Part model, mm, in its own coordinate system. A direction names the side the tool comes from. Coordinates: 2 decimals unless noted, no trailing zeros. Order: outer loops, then holes, each group sorted by start corner. A loop starts at its lowest first (then second) coordinate and runs counter-clockwise, first axis right, second up.
from build123d import *

# Parameters (mm, degrees)
BOSS_EXTRUDE1_DEPTH          = 8
CUT_EXTRUDE1_DEPTH           = 3
F_4_0_4_DIAMETER_HOLE1_D     = 4
F_4_0_4_DIAMETER_HOLE1_DEPTH = 8
FILLET1_R                    = 3
FILLET2_R                    = 5
FILLET3_R                    = 11
FILLET4_R                    = 13


with BuildPart() as part:
    # Sketch1 → Boss-Extrude1 (new body)
    with BuildSketch(Plane.XY.offset(13)):
        with BuildLine():
            Line((-15, 5), (-15, 20))
            ThreePointArc((-15, 20), (-20, 25), (-25, 20))
            Line((-25, 20), (-25, -5))
            Line((-25, -5), (0, -5))
            ThreePointArc((0, -5), (5, 0), (0, 5))
            Line((0, 5), (-15, 5))
        make_face()
    extrude(amount=-BOSS_EXTRUDE1_DEPTH)

    # Sketch2 → Cut-Extrude1 (cut)
    with BuildSketch(Plane.XY.offset(13)):
        with BuildLine():
            Line((-23, 20), (-23, -3))
            Line((-23, -3), (0, -3))
            ThreePointArc((0, -3), (3, 0), (0, 3))
            Line((0, 3), (-17, 3))
            Line((-17, 3), (-17, 20))
            ThreePointArc((-17, 20), (-20, 23), (-23, 20))
        make_face()
    extrude(amount=-CUT_EXTRUDE1_DEPTH, mode=Mode.SUBTRACT)

    # Ø4.0 (4) Diameter Hole1
    with Locations(Plane(origin=(0, 0, 5), x_dir=(-1, 0, 0), z_dir=(0, 0, -1))):
        with Locations((20, 20), (20, 0), (0, 0)):
            Hole(F_4_0_4_DIAMETER_HOLE1_D / 2, depth=F_4_0_4_DIAMETER_HOLE1_DEPTH)

    # Fillet1
    fillet1_edges = [part.edges().sort_by_distance(p)[0] for p in [
        (-23, -3, 11.5),
    ]]
    fillet(fillet1_edges, radius=FILLET1_R)

    # Fillet2
    fillet2_edges = [part.edges().sort_by_distance(p)[0] for p in [
        (-25, -5, 9),
    ]]
    fillet(fillet2_edges, radius=FILLET2_R)

    # Fillet3
    fillet3_edges = [part.edges().sort_by_distance(p)[0] for p in [
        (-15, 5, 9),
    ]]
    fillet(fillet3_edges, radius=FILLET3_R)

    # Fillet4
    fillet4_edges = [part.edges().sort_by_distance(p)[0] for p in [
        (-17, 3, 11.5),
    ]]
    fillet(fillet4_edges, radius=FILLET4_R)


solid = part.part
Q1. Which spindle directions (+Z, -Z, +X, -X, +Y, -Y) get a long thin tool onto all of the face, cutting with end or side? Do faces 5 (the face through (-10, -5, 9)), 6 (the face through (-13.293, 6.909, 11.479)), 7 (the face through (-2, 5, 9)). Say none if no direction does.
Results list:
face 5: +Z, -Z, +X, -X, -Y
face 6: +Z
face 7: +Z, -Z, +X, +Y
Q2. Mould opens along X. For faces 1 (the face through (-16, 7, 10)), 2 (the face through (-14, 7, 5)), 3 (the face through (5, 0, 9)), 4 (the face through (-2, 3, 12)) say: pulls with the +X half, pulls with the -X half, needs draft (parallel to the pull), parting line crosses it, or undercut.
Results list:
face 1: undercut
face 2: needs draft
face 3: pulls with the +X half
face 4: undercut
Q3. Cut at A-A on z = 8.5. Write the cut outline in (x, y).
Results list:
outline: (-25, 0) arc R5 ccw to (-20, -5) - (0, -5) arc R5 ccw to (0, 5) - (-4, 5) arc R11 cw to (-15, 16) - (-15, 20) arc R5 ccw to (-25, 20) - close; hole circle Ø4 at (-20, 0); hole circle Ø4 at (-20, 20); hole circle Ø4 at (0, 0)
Q4. Cut at B-B on x = -19. Write the cut outline in (y, z).
Results list:
outline: (-5, 5) - (-1.73, 5) - (-1.73, 10) - (-3, 10) - (-3, 13) - (-5, 13) - close; (1.73, 5) - (18.27, 5) - (18.27, 10) - (1.73, 10) - close; (21.73, 5) - (24.9, 5) - (24.9, 13) - (22.83, 13) - (22.83, 10) - (21.73, 10) - close
Q5. Cut at D-D on y = 9.5. Write the cut outline in (x, z).
Results list:
outline: (-25, 5) - (-12.87, 5) - (-12.87, 13) - (-15.26, 13) - (-15.26, 10) - (-23, 10) - (-23, 13) - (-25, 13) - close
Q6. Pin check, flat tips, straight feed: pin 1 Ø2.5 at (y, z) = (9.5, 11) entering from +X; pin 2 Ø4.5 at (x, y) = (-20, 20) entering from +Z; pin 3 Ø4.5 at (y, z) = (18, 10) entering from +X. Stop position of each tip, or through.
Results list:
pin 1: stops at x = -11.81
pin 2: stops at z = 10
pin 3: stops at x = -15
Q7. Wall check: line 1 along Y through (x, z) = (-20, 7.9); line 2 along Y through (x, z) = (-1.25, 12.75); line 3 along X through (y, z) = (21.5, 11). Give the ranges that are in metal, low to high.
Results list:
line 1: y = -5 to -2, 2 to 18, 22 to 25
line 2: y = -5 to -3, 3 to 5
line 3: x = -24.77 to -22.6, -17.4 to -15.23
Q8. Cut at C-C on z = 11.75. Write the cut outline in (x, y).
Results list:
outline: (-25, 0) arc R5 ccw to (-20, -5) - (0, -5) arc R5 ccw to (0, 5) - (-4, 5) arc R11 cw to (-15, 16) - (-15, 20) arc R5 ccw to (-25, 20) - close; hole (-23, 0) arc R3 ccw to (-20, -3) - (0, -3) arc R3 ccw to (0, 3) - (-4, 3) arc R13 cw to (-17, 16) - (-17, 20) arc R3 ccw to (-23, 20) - close
